from build123d import *

# Parameters (mm, degrees)
FILLET1_R = 12.7
FILLET2_R = 6.35


with BuildPart() as part:
    # Sketch1 → Revolve1 (revolve)
    with BuildSketch(Plane.XY):
        Polygon((-0.381, -44.3484), (13.568194302, -27.724397577), (16.383, -30.0863), (51.181, -30.3149), (51.181, -34.417), (15.412836736, -34.417), (2.028190699, -50.3682), (-51.181, -50.3682), (-51.181, -44.6532), align=None)
    revolve(axis=Axis((-51.181, 0, 0), (1, 0, 0)))

    # Fillet1
    fillet1_edges = [part.edges().sort_by_distance(p)[0] for p in [
        (2.028190699, 50.3682, 0),
    ]]
    fillet(fillet1_edges, radius=FILLET1_R)

    # Fillet2
    fillet2_edges = [part.edges().sort_by_distance(p)[0] for p in [
        (15.412836736, 34.417, 0),
    ]]
    fillet(fillet2_edges, radius=FILLET2_R)


solid = part.part
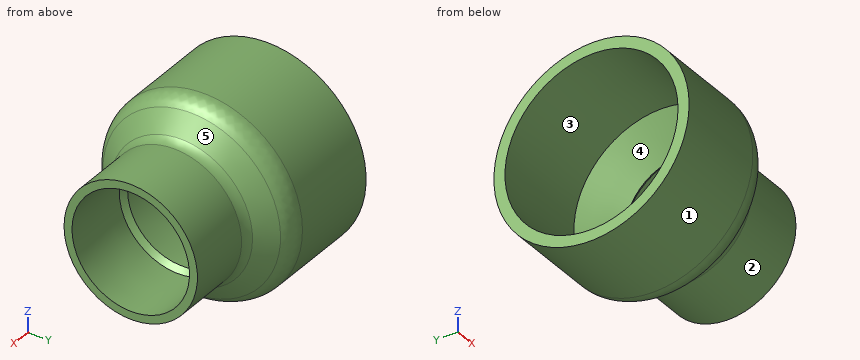
Check sheet for the modelled part. Datum: model origin and axes. Units: mm. Face numbers are marked on the shaded views. A direction names the side the tool comes from. Round coordinates to 2 decimals unless told otherwise and drop trailing zeros. Order: outer loops, then holes, each group sorted by start corner. A loop starts at its lowest first (then second) coordinate and runs counter-clockwise, first axis right, second up.
(1) Draft check along Y on the marked faces 4 and 5. Enter one of: pulls with the +Y half, pulls with the -Y half, needs draft (parallel to the pull), parting line crosses it, or undercut.
(2) Go/stop test with flat-tipped pins: P1, Ø6, axis at y = 7, z = 35.5, coming from the -X side; P2, Ø12, axis at x = -23, z = 5, coming from the -Y side; P3, Ø8, axis at x = 21, y = -13, coming from the +Z side; P4, Ø4, axis at x = -22.5, y = 39, coming from the +Z side. Record where each tip stops, or that it passes through.
(3) Cross-section at B-B, the plane x = 43.5. Enter the section's corners in (y, z), and give its area (3 significant figures).
(4) Cross-section at A-A, the plane x = -6. Enter the section's corners in (y, z), and give its area (3 significant figures).
(5) Access from +Z, -Z, +X, -X, +Y, -Y to the whole of each face (thin tool, end or side, straight path). Record for the marked faces 1, 2 and 3.
(6) Scan lines: probe 1 along Z at (x, y) = (25, -1); probe 2 along Z at (x, y) = (-33, -39); probe 3 along Y at (x, z) = (45.5, -1). Record each from-to range of solid material in increasing order.
Check sheet entries:
1. face 4: undercut
1. face 5: parting line crosses it
2. P1: stops at x = 3.95
2. P2: stops at y = -50.37
2. P3: stops at z = 33.22
2. P4: stops at z = 34.18
3. outline: circle Ø68.83 at (0, 0); hole circle Ø60.53 at (0, 0)
3. area: 844 mm2
4. outline: circle Ø100.74 at (0, 0); hole circle Ø88.76 at (0, 0)
4. area: 1,780 mm2
5. face 1: +X, -X
5. face 2: +X
5. face 3: -X
6. probe 1: z = -34.4 to -30.13, 30.13 to 34.4
6. probe 2: z = -31.87 to -21.52, 21.52 to 31.87
6. probe 3: y = -34.4 to -30.26, 30.26 to 34.4
